```python
from build123d import *

# Parameters (mm, degrees)
SKETCH1_W             = 0.34
SKETCH1_H             = 2.75
BOSS_EXTRUDE1_DEPTH   = 1.25
SKETCH1_W_2           = 0.339999955
BOSS_EXTRUDE1_2_DEPTH = 1.25
BOSS_EXTRUDE2_DEPTH   = 2.75


with BuildPart() as part:
    # Sketch1 → Boss-Extrude1 (new body)
    with BuildSketch(Plane.XY):
        with Locations((-0.17, 1.375)):
            Rectangle(SKETCH1_W, SKETCH1_H)
    extrude(amount=BOSS_EXTRUDE1_DEPTH)



with BuildPart() as body_2:
    # Sketch1 → Boss-Extrude1 2 (new body)
    with BuildSketch(Plane.XY):
        with Locations((15.759999978, 1.375)):
            Rectangle(SKETCH1_W_2, SKETCH1_H)
    extrude(amount=BOSS_EXTRUDE1_2_DEPTH)


with BuildPart() as part_1:
    add(part.part)

    add(body_2.part)  # Boss-Extrude2 merges body 2
    # Sketch2 → Boss-Extrude2 (add)
    with BuildSketch(Plane(origin=(0, 2.75, 0), x_dir=(1, 0, 0), z_dir=(0, 1, 0))):
        with BuildLine():
            Line((-0.339999955, -1.25), (0, -1.25))
            ThreePointArc((0, -1.25), (7.795, -9.045), (15.59, -1.25))
            Line((15.59, -1.25), (15.929999955, -1.25))
            ThreePointArc((15.929999955, -1.25), (7.795, -11.627244432), (-0.339999955, -1.25))
        make_face()
    extrude(amount=-BOSS_EXTRUDE2_DEPTH)


solid = part_1.part
```
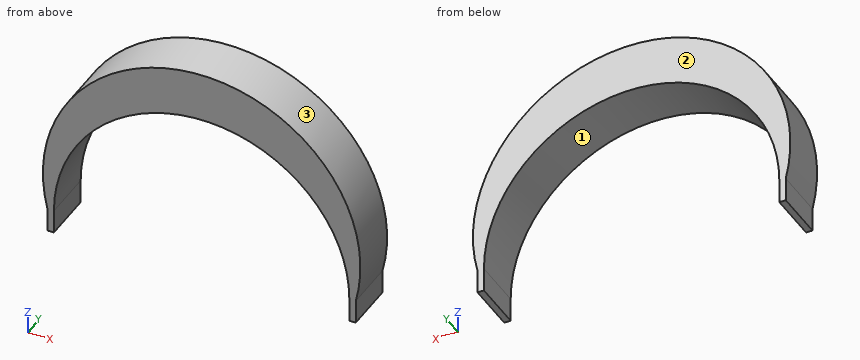
Here's how the part is built. I have some questions about the finished solid (model axes, mm). Face numbers are marked on the shaded views. Coordinates: 2 decimals unless noted, no trailing zeros. Order: outer loops, then holes, each group sorted by start corner. A loop starts at its lowest first (then second) coordinate and runs counter-clockwise, first axis right, second up.
Item 1: If we section it at D-D, the plane x = 6.25: List the corners of the cut face in (y, z) for me, then the cut area to 3 significant figures.
Response values:
outline: (0, 8.89) - (2.75, 8.89) - (2.75, 11.48) - (0, 11.48) - close
area: 7.13 mm2
Item 2: If we section it at B-B, the plane y = 1.85: List the corners of the cut face in (x, z) for me (3 decimals), then the cut area to 3 significant figures.
Response values:
outline: (-0.34, 0) - (0, 0) - (0, 1.25) arc R7.795 cw to (15.59, 1.25) - (15.59, 0) - (15.93, 0) - (15.93, 1.25) arc R8.377 ccw (long way) to (-0.34, 1.25) - close
area: 48.8 mm2
Item 3: If we section it at A-A, the plane z = 5.5: List the corners of the cut face in (x, y) for me, then the cut area to 3 significant figures.
Response values:
outline: (-0.27, 0) - (1.26, 0) - (1.26, 2.75) - (-0.27, 2.75) - close; (14.33, 0) - (15.86, 0) - (15.86, 2.75) - (14.33, 2.75) - close
area: 8.44 mm2
Item 4: If we section it at C-C, the plane z = 6.75: List the corners of the cut face in (x, y) for me, then the cut area to 3 significant figures.
Response values:
outline: (0.18, 0) - (2.27, 0) - (2.27, 2.75) - (0.18, 2.75) - close; (13.32, 0) - (15.41, 0) - (15.41, 2.75) - (13.32, 2.75) - close
area: 11.5 mm2
Item 5: I need wall thicknesses on probe 1 along X at (y, z) = (1.55, 3.5); probe 2 along X at (y, z) = (1.45, 4); probe 3 along Z at (x, y) = (10.5, 0.9). Which ranges of each line are inside material? Lowest first, please.
Response values:
probe 1: x = -0.58 to 0.33, 15.26 to 16.17
probe 2: x = -0.55 to 0.5, 15.09 to 16.14
probe 3: z = 8.56 to 11.18
Item 6: Thinking about a two-plate mould opening in X: for the marked faces 1, 2 and 3, which applies, pulls with the +X half, pulls with the -X half, needs draft (parallel to the pull), parting line crosses it, or undercut?
Response values:
face 1: undercut
face 2: needs draft
face 3: parting line crosses it
Item 7: I'm going to push flat-ended pins straight in: pin 1 Ø1.4 at (y, z) = (0.5, 0.5) entering from -X; pin 2 Ø1.5 at (y, z) = (2, 2) entering from +X. Where does each tip first touch, or does it pass through?
Response values:
pin 1: stops at x = -0.34
pin 2: stops at x = 16.16
